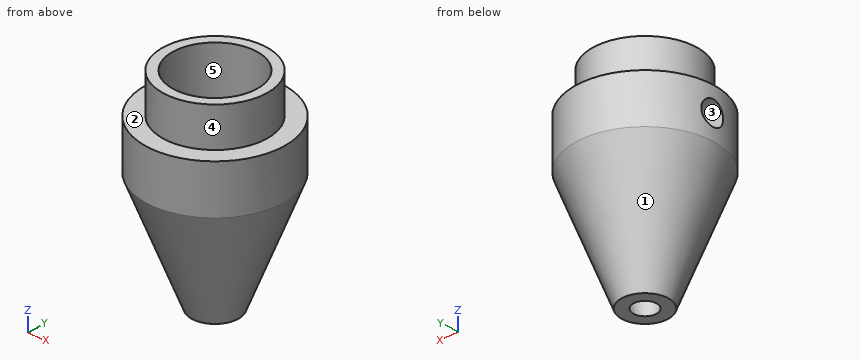
from build123d import *

# Parameters (mm, degrees)
F0_R      = 9.335
F1_DEPTH  = 7
F2_R      = 12.425
F2_R_2    = 9.335
F3_DEPTH  = 8.7
F3_FACE_R = 12.425
F5_R      = 4.2
F8_R      = 7.57
F10_DEPTH = 15.7
F11_R     = 7.57
F9_R      = 2.1
F13_R     = 2.15
F14_REACH = 30.9321184182


with BuildPart() as f1:
    # F0 (on Top) → F1 (new body)
    with BuildSketch(Plane.XY):
        Circle(F0_R)
    extrude(amount=-F1_DEPTH)

    # F2 (on face) → F3 (join)
    with BuildSketch(Plane(origin=(0, 0, -7), x_dir=(1, 0, 0), z_dir=(0, 0, -1))):
        Circle(F2_R)
        Circle(F2_R_2, mode=Mode.SUBTRACT)
        Circle(F2_R_2)
    extrude(amount=F3_DEPTH)

    # F3_face (on face) → F6 section 0
    with BuildSketch(Plane(origin=(0, 0, -15.7), x_dir=(1, 0, 0), z_dir=(0, 0, -1))):
        Circle(F3_FACE_R)
    # F5 (on offset) → F6 section 1
    with BuildSketch(Plane(origin=(0, 0, -36.675), x_dir=(1, 0, 0), z_dir=(0, 0, -1))):
        Circle(F5_R)
    loft()

    # F8 (on face) → F10 (cut)
    with BuildSketch(Plane.XY):
        Circle(F8_R)
    extrude(amount=-F10_DEPTH, mode=Mode.SUBTRACT)

    # F11 (on face) → F12 section 0
    with BuildSketch(Plane.XY.offset(-15.7)):
        Circle(F11_R)
    # F9 (on face) → F12 section 1
    with BuildSketch(Plane(origin=(0, 0, -36.675), x_dir=(1, 0, 0), z_dir=(0, 0, -1))):
        Circle(F9_R)
    loft(mode=Mode.SUBTRACT)

    f14_end = f1.faces().sort_by_distance((-7.57, 0, -7.85))[0]
    # F13 (on offset) → F14 (cut, up to a face of the model that its end follows)
    with BuildSketch(Plane.YZ.offset(-12.425)):
        with Locations((0, -11.35)):
            Circle(F13_R)
    f14_long = extrude(amount=F14_REACH, mode=Mode.PRIVATE)
    add(split(f14_long, bisect_by=f14_end, keep=Keep.ALL, mode=Mode.PRIVATE).solids().sort_by_distance((-12.425, 0, -11.35))[0], mode=Mode.SUBTRACT)


solid = f1.part
Work out the finished part from the listing and answer in its coordinate system (mm). Face numbers are marked on the shaded views. A direction names the side the tool comes from. Coordinates: 2 decimals unless noted, no trailing zeros. Order: outer loops, then holes, each group sorted by start corner. A loop starts at its lowest first (then second) coordinate and runs counter-clockwise, first axis right, second up. Notation, with made-up numbers: (-30, 71.25) - (12, 71.25) arc R28 cw to (12, 93.25) - close; hole circle Ø4 at (8, 29). An arc over 180 degrees is marked (long way). Put each result on its own line as item: value. Start each with the question number.
1) Find section A-A (x = 0). Give the vertices of the cut face in (y, z) (3 decimals).
2) Find section B-B (y = 0). State how many separate pieces and enclosed holes the cut face has, plus the area to 3 significant figures.
3) Flat-ended cylindrical pins translate along their axes: pin 1 (2 mm diameter, centred on x = -3, z = -8, fed in from -Y); pin 2 (2 mm diameter, centred on x = 4, z = -13, fed in from -Y); pin 3 (3 mm diameter, centred on x = 8, z = -24.5, fed in from +Y). Find the tip coordinate at first contact, or state that the pin passes through.
4) Find the intervals of material crossed by line 1 (X direction, y = 0, z = -8.5) (3 decimals); line 2 (Y direction, x = 3.5, z = -21.5), in increasing order. Write a range as from..to.
5) Find section C-C (z = -30). Give the vertices of the cut face in (x, y).
6) For a pull along X with two mould halves and no side action, classify the marked faces 3, 4 and 5 as released by +X, released by -X, zero draft, split by the parting line, or undercut.
7) For the marked faces 1 and 2, determine the directions among +Z, -Z, +X, -X, +Y, -Y from which every point of the face is accessible in a straight line to the end or side of a thin tool.
8) Find section D-D (z = -11.35). Give the vertices of the cut face in (x, y) (3 decimals).
Results list:
1. outline: (-12.425, -15.7) - (-4.2, -36.675) - (-2.1, -36.675) - (-7.57, -15.7) - (-7.57, 0) - (-9.335, 0) - (-9.335, -7) - (-12.425, -7) - close; (2.1, -36.675) - (4.2, -36.675) - (12.425, -15.7) - (12.425, -7) - (9.335, -7) - (9.335, 0) - (7.57, 0) - (7.57, -15.7) - close
2. separate pieces: 3
2. enclosed holes: 0
2. area: 234 mm^2
3. pin 1: stops at y = -12.26
3. pin 2: stops at y = -12.06
3. pin 3: stops at y = 6.4
4. line 1: x = -12.425..-7.57, 7.57..12.425
4. line 2: y = -9.53..-4.94, 4.94..9.53
5. outline: circle Ø13.63 at (0, 0); hole circle Ø7.68 at (0, 0)
6. face 3: zero draft
6. face 4: split by the parting line
6. face 5: undercut
7. face 1: -Z
7. face 2: +Z
8. outline: (-12.238, -2.15) arc R12.425 ccw (long way) to (-12.238, 2.15) - (-7.258, 2.15) arc R7.57 cw (long way) to (-7.258, -2.15) - close
